from build123d import *

# Parameters (mm, degrees)
BOSS_EXTRUDE1_DEPTH = 33.274
HOLE1_D             = 8.3312
HOLE1_DEPTH         = 6.35
HOLE2_D             = 8.3312
HOLE2_DEPTH         = 6.35
FILLET1_R           = 7.9248


with BuildPart() as part:
    # Sketch1 → Boss-Extrude1 (new body)
    with BuildSketch(Plane(origin=(16.637, 0, 0), x_dir=(0, 0, -1), z_dir=(1, 0, 0))):
        with BuildLine():
            Line((-38.1, 0), (0, 0))
            Line((0, 0), (0, 38.1))
            ThreePointArc((0, 38.1), (-4.490128061, 36.240128061), (-6.35, 31.75))
            Line((-6.35, 31.75), (-6.35, 6.35))
            Line((-6.35, 6.35), (-31.75, 6.35))
            ThreePointArc((-31.75, 6.35), (-36.240128061, 4.490128061), (-38.1, 0))
        make_face()
    extrude(amount=-BOSS_EXTRUDE1_DEPTH)

    # Hole1
    with Locations(Plane.XY.offset(6.35)):
        with Locations((0, 19.05)):
            Hole(HOLE1_D / 2, depth=HOLE1_DEPTH)

    # Hole2
    with Locations(Plane(origin=(0, 6.35, 0), x_dir=(1, 0, 0), z_dir=(0, 1, 0))):
        with Locations((0, -19.05)):
            Hole(HOLE2_D / 2, depth=HOLE2_DEPTH)

    # Fillet1
    fillet1_edges = [part.edges().sort_by_distance(p)[0] for p in [
        (0, 6.35, 6.35),
    ]]
    fillet(fillet1_edges, radius=FILLET1_R)


solid = part.part
Geometry check sheet. Reference: the model listing, model coordinates, mm. A direction names the side the tool comes from. Round coordinates to 2 decimals unless told otherwise and drop trailing zeros. Write each loop counter-clockwise with the first axis right and the second up, starting at its lowest first coordinate (ties: lowest second). Pieces come first, ordered by that corner, then holes. Notation, with made-up numbers: (-9, -16.75) -> (30, -16.75) arc R21 ccw to (30, 5.25) -> close; hole circle Ø5 at (-28, 82). An arc over 180 degrees is marked (long way). One line per item, written item: value. Start each with the question number.
(1) Access from +Z, -Z, +X, -X, +Y, -Y to the whole of each face (thin tool, end or side, straight path). Record for faces 1 (the flat face through (0, 6.35, 25)), 2 (the flat face through (0, 0, 24)).
(2) Cross-section at A-A, the plane y = 19.05. Record the cut outline in (x, z).
(3) Scan lines: line 1 (X direction, y = 5, z = 19.05); line 2 (Y direction, x = -4.5, z = 31.5). Record each from-to range of solid material in increasing order. Write a range as [from, to].
(4) Cross-section at C-C, the plane x = -8. Record the cut outline in (y, z).
(5) Go/stop test with flat-tipped pins: pin 1 Ø5 at (x, z) = (4, 17) entering from +Y; pin 2 Ø14 at (x, y) = (6.5, 24.5) entering from +Z. Record where each tip stops, or that it passes through.
(6) Draft check along Z on faces 3 (the cylindrical face through (0.54, 3.13, 14.92)), 4 (the flat face through (16.637, 6, 11)), 5 (the cylindrical face through (0.23, 36.29, 4.44)), 6 (the flat face through (0.2, 14.5, 0)). Enter one of: +Z half, -Z half, draft (parallel to the pull), parting line (faces both ways), or undercut.
(7) Cross-section at D-D, the plane x = 0. Record the cut outline in (y, z), and give its area (3 significant figures).
Answer:
1. face 1: +Z, +X, -X, +Y
1. face 2: +Z, -Z, +X, -X, -Y
2. outline: (-16.64, 0) -> (-4.17, 0) -> (-4.17, 6.35) -> (-16.64, 6.35) -> close; (4.17, 0) -> (16.64, 0) -> (16.64, 6.35) -> (4.17, 6.35) -> close
3. line 1: [-16.64, -4.17], [4.17, 16.64]
3. line 2: [0, 6.35]
4. outline: (0, 0) -> (38.1, 0) arc R6.35 ccw to (31.75, 6.35) -> (14.27, 6.35) arc R7.92 cw to (6.35, 14.27) -> (6.35, 31.75) arc R6.35 ccw to (0, 38.1) -> close
5. pin 1: y = 6.35
5. pin 2: z = 6.35
6. face 3: undercut
6. face 4: draft
6. face 5: +Z half
6. face 6: -Z half
7. outline: (0, 0) -> (14.88, 0) -> (14.88, 6.35) -> (14.27, 6.35) arc R7.92 cw to (6.35, 14.27) -> (6.35, 14.88) -> (0, 14.88) -> close; (0, 23.22) -> (6.35, 23.22) -> (6.35, 31.75) arc R6.35 ccw to (0, 38.1) -> close; (23.22, 0) -> (38.1, 0) arc R6.35 ccw to (31.75, 6.35) -> (23.22, 6.35) -> close
7. area: 334 mm²
